Part model, mm, in its own coordinate system. Face numbers are marked on the shaded views. A direction names the side the tool comes from. Coordinates: 2 decimals unless noted, no trailing zeros. Loops run counter-clockwise (first coordinate to the right, second up) from the corner with the lowest first, then second, coordinate; pieces in that order, holes last. Notation, with made-up numbers: (-1, 31.5) - (56, 31.5) arc R22 ccw to (56, 67.5) - close; hole circle Ø10 at (2.5, 67). An arc over 180 degrees is marked (long way). Use a Markdown table: item, result. Add a question column.
1. Band-saw the part on A-A, the plane x = -16. Give the cut face in (y, z).
2. Band-saw the part on C-C, the plane z = 11. Give the cut face in (x, y).
3. Pull direction X, two halves, no side cores. Call the marked faces 1, 2 and 3: pulls with the +X half, pulls with the -X half, needs draft (parallel to the pull), parting line crosses it, or undercut.
4. Band-saw the part on B-B, the plane y = 23. Give the cut face in (x, z).
5. Drop flat-ended pins along their axis: pin 1 (7 mm diameter, centred on y = 31, z = 3.5, fed in from +X); pin 2 (6 mm diameter, centred on x = 0, y = 31.5, fed in from +Z); pin 3 (4 mm diameter, centred on y = 28.5, z = 4.5, fed in from -X); pin 4 (3.5 mm diameter, centred on y = 33, z = 7.5, fed in from -X). Give the stop position or say it passes through.
6. 3-axis set-ups, long thin cutter, end or side, ignore diameter. For the marked faces 4, 5 and 6: which of +Z, -Z, +X, -X, +Y, -Y reach the whole face in a straight line?
7. Wall check: probe 1 along X at (y, z) = (4.2, 7); probe 2 along Y at (x, z) = (9.2, 7); probe 3 along X at (y, z) = (23, 5.5). Give the ranges that are in metal, low to high. Write a range as [from, to].
8. Band-saw the part on D-D, the plane x = 0. Give the cut face in (y, z).
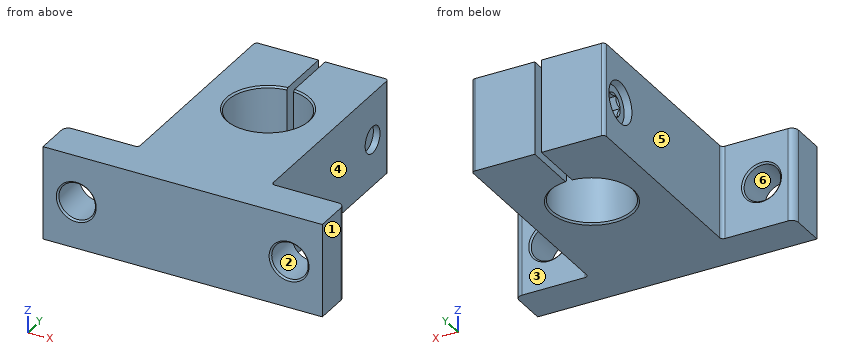
from build123d import *

# Parameters (mm, degrees)
BOSS_EXTRUDE1_DEPTH     = 14
CUT_EXTRUDE1_DEPTH      = 46.202322949
CUT_EXTRUDE1_DEPTH_BACK = 6
SKETCH3_R               = 2.75
FILLET1_R               = 1
FILLET2_R               = 0.5
CHAMFER1_SIZE           = 0.25
SKETCH4_R               = 3.1
CUT_EXTRUDE2_DEPTH      = 1
SKETCH5_R               = 3.1
SKETCH5_R_2             = 3
CUT_EXTRUDE3_DEPTH      = 4
CHAMFER2_SIZE           = 0.2
CUT_EXTRUDE4_DEPTH      = 2
SKETCH7_R               = 2
BOSS_EXTRUDE2_DEPTH     = 1
CUT_EXTRUDE5_START      = -1
SKETCH8_R               = 2
CUT_EXTRUDE5_DEPTH      = 1
SKETCH9_R               = 1.732050808
CUT_EXTRUDE6_DEPTH      = 1
CUT_EXTRUDE6_DRAFT      = -45


with BuildPart() as part:
    # Sketch1 → Boss-Extrude1 (new body)
    with BuildSketch(Plane.XY):
        with BuildLine():
            Line((-21, 0), (21, 0))
            Line((21, 0), (21, 6))
            Line((21, 6), (10, 6))
            Line((10, 6), (10, 37.5))
            Line((10, 37.5), (0.5, 37.5))
            Line((0.5, 37.5), (0.5, 28.979130372))
            ThreePointArc((0.5, 28.979130372), (0, 17), (-0.5, 28.979130372))
            Line((-0.5, 28.979130372), (-0.5, 37.5))
            Line((-0.5, 37.5), (-10, 37.5))
            Line((-10, 37.5), (-10, 6))
            Line((-10, 6), (-21, 6))
            Line((-21, 6), (-21, 0))
        make_face()
    extrude(amount=BOSS_EXTRUDE1_DEPTH)

    # Sketch3 → Cut-Extrude1 (cut, two sides: drawn at the far end of the back side and taken through both)
    with BuildSketch(Plane.XZ.offset(-CUT_EXTRUDE1_DEPTH_BACK)):
        with Locations(Location((-16, 7, 0), (0, 0, 180))):
            Circle(SKETCH3_R)
        with Locations(Location((16, 7, 0), (0, 0, 180))):
            Circle(SKETCH3_R)
    extrude(amount=CUT_EXTRUDE1_DEPTH + CUT_EXTRUDE1_DEPTH_BACK, mode=Mode.SUBTRACT)

    # Fillet1
    fillet1_edges = [part.edges().sort_by_distance(p)[0] for p in [
        (-21, 6, 7),
        (21, 6, 7),
    ]]
    fillet(fillet1_edges, radius=FILLET1_R)

    # Fillet2
    fillet2_edges = [part.edges().sort_by_distance(p)[0] for p in [
        (-10, 6, 7),
        (-10, 37.5, 7),
        (10, 37.5, 7),
        (10, 6, 7),
    ]]
    fillet(fillet2_edges, radius=FILLET2_R)

    # Chamfer1
    chamfer1_edges = [part.edges().sort_by_distance(p)[0] for p in [
        (0, 17, 0),
        (0, 17, 14),
        (18.75, 6, 7),
        (18.75, 0, 7),
        (-13.25, 6, 7),
        (-13.25, 0, 7),
    ]]
    chamfer(chamfer1_edges, length=CHAMFER1_SIZE)

    # Sketch4 → Cut-Extrude2 (cut)
    with BuildSketch(Plane.ZY.offset(10)):
        with Locations(Location((7, 33.25, 0), (0, 0, 270))):
            Circle(SKETCH4_R)
    extrude(amount=-CUT_EXTRUDE2_DEPTH, mode=Mode.SUBTRACT)

    # Sketch5 → Cut-Extrude3 (cut)
    with BuildSketch(Plane.ZY.offset(9)):
        with Locations(Location((7, 33.25, 0), (0, 0, 270))):
            Circle(SKETCH5_R)
        with Locations(Location((7, 33.25, 0), (0, 0, 270))):
            Circle(SKETCH5_R_2, mode=Mode.SUBTRACT)
    extrude(amount=-CUT_EXTRUDE3_DEPTH, mode=Mode.SUBTRACT)

    # Chamfer2
    chamfer2_edges = [part.edges().sort_by_distance(p)[0] for p in [
        (-9, 36.25, 7),
    ]]
    chamfer(chamfer2_edges, length=CHAMFER2_SIZE)

    # Sketch6 → Cut-Extrude4 (cut)
    with BuildSketch(Plane.ZY.offset(9)):
        Polygon((7.246062581, 31.535516636), (8.607817438, 32.605854763), (8.361754858, 34.320338128), (6.753937419, 34.964483364), (5.392182562, 33.894145237), (5.638245142, 32.179661872), align=None)
    extrude(amount=-CUT_EXTRUDE4_DEPTH, mode=Mode.SUBTRACT)

    # Sketch7 → Boss-Extrude2 (add)
    with BuildSketch(Plane(origin=(-0.5, 0, 0), x_dir=(0, 0, -1), z_dir=(1, 0, 0))):
        with Locations(Location((-7, 33.25, 0), (0, 0, 270))):
            Circle(SKETCH7_R)
    extrude(amount=BOSS_EXTRUDE2_DEPTH)

    # Sketch8 → Cut-Extrude5 (cut)
    with BuildSketch(Plane(origin=(10, 0, 0), x_dir=(0, 0, -1), z_dir=(1, 0, 0)).offset(CUT_EXTRUDE5_START)):
        with Locations(Location((-7, 33.25, 0), (0, 0, 270))):
            Circle(SKETCH8_R)
    extrude(amount=CUT_EXTRUDE5_DEPTH, mode=Mode.SUBTRACT)


with BuildPart() as cut_extrude6_tool:
    # Sketch9 → Cut-Extrude6 (with draft: the straight prism first)
    with BuildSketch(Plane.ZY.offset(9)):
        with Locations((7, 33.25)):
            Circle(SKETCH9_R)
    extrude(amount=-CUT_EXTRUDE6_DEPTH)
    # Cut-Extrude6: the draft: its side faces are tilted about the plane it starts from
    cut_extrude6_sides = [cut_extrude6_tool.faces().sort_by_distance(p)[0] for p in [
        (-8.5, 33.25, 5.267949192),
    ]]
    draft(cut_extrude6_sides, Plane.ZY.offset(9), CUT_EXTRUDE6_DRAFT)


with BuildPart() as part_1:
    add(part.part)

    # Cut-Extrude6: cut by cut_extrude6_tool
    add(cut_extrude6_tool.part, mode=Mode.SUBTRACT)


solid = part_1.part
Geometry check:
| question | item | result |
|---|---|---|
| 1 | outline | (0, 0) - (6, 0) - (6, 4) - (5.75, 4.25) - (0.25, 4.25) - (0, 4) - close; (0, 10) - (0.25, 9.75) - (5.75, 9.75) - (6, 10) - (6, 14) - (0, 14) - close |
| 2 | outline | (-21, 0) - (21, 0) - (21, 5) arc R1 ccw to (20, 6) - (10.5, 6) arc R0.5 cw to (10, 6.5) - (10, 37) arc R0.5 ccw to (9.5, 37.5) - (0.5, 37.5) - (0.5, 28.98) arc R6 cw (long way) to (-0.5, 28.98) - (-0.5, 37.5) - (-9.5, 37.5) arc R0.5 ccw to (-10, 37) - (-10, 6.5) arc R0.5 cw to (-10.5, 6) - (-20, 6) arc R1 ccw to (-21, 5) - close |
| 3 | face 1 | pulls with the +X half |
| 3 | face 2 | undercut |
| 3 | face 3 | needs draft |
| 4 | outline | (-10, 0) - (-6.25, 0) - (-6, 0.25) - (-6, 13.75) - (-6.25, 14) - (-10, 14) - close; (6, 0.25) - (6.25, 0) - (10, 0) - (10, 14) - (6.25, 14) - (6, 13.75) - close |
| 5 | pin 1 | stops at x = 10 |
| 5 | pin 2 | stops at z = 14 |
| 5 | pin 3 | stops at x = -10 |
| 5 | pin 4 | stops at x = -9 |
| 6 | face 4 | +Z, -Z, +X, +Y |
| 6 | face 5 | +Z, -Z, -X, +Y |
| 6 | face 6 | +Y, -Y |
| 7 | probe 1 | x = [-21, -18.75], [-13.25, 13.25], [18.75, 21] |
| 7 | probe 2 | y = [0, 31.25], [35.25, 37.5] |
| 7 | probe 3 | x = [-10, -6], [6, 10] |
| 8 | outline | (0, 0) - (16.75, 0) - (17, 0.25) - (17, 13.75) - (16.75, 14) - (0, 14) - close; circle Ø4 at (33.25, 7) |
